Verification items for the finished model (mm, model axes). A direction names the side the tool comes from. Coordinates: 2 decimals unless noted, no trailing zeros. Order: outer loops, then holes, each group sorted by start corner. A loop starts at its lowest first (then second) coordinate and runs counter-clockwise, first axis right, second up. Notation, with made-up numbers: M 26,36 L 63,36 A11 ccw 63,56 Z; hole C 67.25,-38 d11. An arc over 180 degrees is marked long. Answer as a JSON object with one key per item and string values. Group by question number.
(1) Mould release check, pull along X, two halves, no side actions. Record for faces 3 (the face through (1, -2, 15)), 4 (the face through (-45, 0, 1)), 5 (the face through (-46, -2, 2)), 6 (the face through (46, -2, -2)): released by +X, released by -X, zero draft, split by the parting line, or undercut.
(2) Cross-section at A-A (z = 31). Enter the section's corners in (x, y), plus the area to 3 significant figures.
(3) Access from +Z, -Z, +X, -X, +Y, -Y to the whole of each face (thin tool, end or side, straight path). Record for faces 1 (the face through (1, -2, 125)), 2 (the face through (-42, -2, 46)).
(4) Material ranges on line 1 (X direction, y = -0.3, z = 81.5); line 2 (Z direction, x = 5, y = -1.25); line 3 (X direction, y = -2.65, z = 57), recorded low to high.
(5) Cross-section at B-B (x = 36). Enter the section's corners in (y, z).
(6) Cross-section at C-C (y = -3.3). Count the separate pieces of the cut face and the enclosed holes in it, plus the area to 3 significant figures.
from build123d import *

# Parameters (mm, degrees)
F0_W     = 2
F0_H     = 40
F0_W_2   = 42
F0_H_2   = 4
F1_DEPTH = 4


with BuildPart() as f1:
    # F0 (on Front) → F1 (new body)
    with BuildSketch(Plane.XZ):
        Polygon((-46, 125), (-46, 0), (-42, 0), (-42, 11), (-42, 15), (-42, 77), (-42, 81), (-42, 121), (-42, 125), align=None)
        Polygon((-42, 0), (-46, 0), (-46, -125), (-42, -125), (-42, -121), (-42, -89), (-42, -81), (-42, -77), (-42, -15), (-42, -11), align=None)
        Polygon((0, 125), (-42, 125), (-42, 121), (-2, 121), (0, 121), align=None)
        Polygon((-42, -121), (-42, -125), (0, -125), (0, -121), (-2, -121), align=None)
        Polygon((42, 11), (42, 0), (46, 0), (46, 125), (42, 125), (42, 121), (42, 81), (42, 77), (42, 15), align=None)
        Polygon((46, 0), (42, 0), (42, -11), (42, -15), (42, -77), (42, -81), (42, -121), (42, -125), (46, -125), align=None)
        Polygon((42, 125), (0, 125), (0, 121), (2, 121), (42, 121), align=None)
        Polygon((0, -121), (0, -125), (42, -125), (42, -121), (2, -121), align=None)
        Polygon((0, -77), (-42, -77), (-42, -81), (-2, -81), (0, -81), align=None)
        Polygon((42, -77), (0, -77), (0, -81), (2, -81), (42, -81), align=None)
        Polygon((-2, -113), (-2, -121), (0, -121), (0, -81), (-2, -81), align=None)
        with Locations((1, -101)):
            Rectangle(F0_W, F0_H)
        with Locations((-21, -13)):
            Rectangle(F0_W_2, F0_H_2)
        with Locations((21, -13)):
            Rectangle(F0_W_2, F0_H_2)
        with Locations((21, 13)):
            Rectangle(F0_W_2, F0_H_2)
        with Locations((-21, 13)):
            Rectangle(F0_W_2, F0_H_2)
        Polygon((-42, 81), (-42, 77), (0, 77), (0, 81), (-2, 81), align=None)
        Polygon((0, 81), (0, 77), (42, 77), (42, 81), (2, 81), align=None)
        with Locations((1, 101)):
            Rectangle(F0_W, F0_H)
        with Locations((-1, 101)):
            Rectangle(F0_W, F0_H)
    extrude(amount=F1_DEPTH)


solid = f1.part
Taken from the geometry:
{
 "1": {"face 3": "undercut", "face 4": "zero draft", "face 5": "released by -X", "face 6": "released by +X"},
 "2": {"outline": "M -46,-4 L -42,-4 L -42,0 L -46,0 Z; M 42,-4 L 46,-4 L 46,0 L 42,0 Z", "area": "32.0 mm²"},
 "3": {"face 1": "+Z, +X, -X, +Y, -Y", "face 2": "+Y, -Y"},
 "4": {"line 1": "x = -46 to -42, -2 to 2, 42 to 46", "line 2": "z = -125 to -121, -81 to -77, -15 to -11, 11 to 15, 77 to 81, 121 to 125", "line 3": "x = -46 to -42, 42 to 46"},
 "5": {"outline": "M -4,-125 L 0,-125 L 0,-121 L -4,-121 Z; M -4,-81 L 0,-81 L 0,-77 L -4,-77 Z; M -4,-15 L 0,-15 L 0,-11 L -4,-11 Z; M -4,11 L 0,11 L 0,15 L -4,15 Z; M -4,77 L 0,77 L 0,81 L -4,81 Z; M -4,121 L 0,121 L 0,125 L -4,125 Z"},
 "6": {"separate pieces": "1", "enclosed holes": "7", "area": "4,340 mm²"}
}
